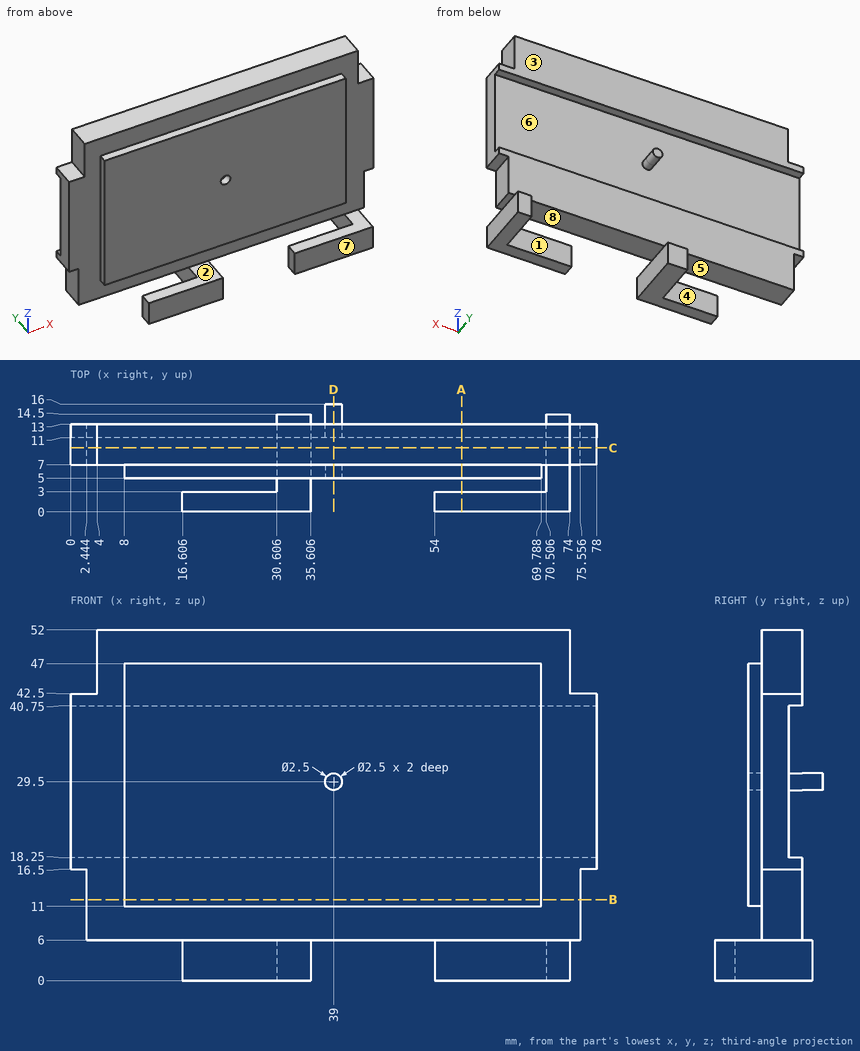
Verification items for this drawing (mm, ordinates from the low corner). A direction names the side the tool comes from. Coordinates: 2 decimals unless noted, no trailing zeros. Write each loop counter-clockwise with the first axis right and the second up, starting at its lowest first coordinate (ties: lowest second). Pieces come first, ordered by that corner, then holes. Notation, with made-up numbers: (-17.5, -0.75) -> (-5.5, -0.75) arc R15 ccw to (-5.5, 21.25) -> close; hole circle Ø11 at (18.5, -36.75). An arc over 180 degrees is marked (long way). One line per item, written item: value. Start each with the question number.
Q1. Cross-section at B-B on z = 12. Enter the section's corners in (x, y) (1 decimal), and give its area (3 significant figures).
Q2. Thickness scan on L1, parallel to Z at x = 54.5, y = 11.25; L2, parallel to Z at x = 39, y = 5.8; L3, parallel to Z at x = 58, y = 6. Record the ranges inside material, lowest first. Write a range as from..to.
Q3. Access from +Z, -Z, +X, -X, +Y, -Y to the whole of each face (thin tool, end or side, straight path). Record for the marked faces 1, 2, 3, 4 and 5.
Q4. Cross-section at D-D on x = 39. Enter the section's corners in (y, z).
Q5. Mould release check, pull along Z, two halves, no side actions. Record for the marked faces 6, 7 and 8: pulls with the +Z half, pulls with the -Z half, needs draft (parallel to the pull), parting line crosses it, or undercut.
Q6. Cross-section at A-A on x = 58. Enter the section's corners in (y, z).
Q7. Cross-section at C-C on y = 9.5. Enter the section's corners in (x, z) (1 decimal), and give its area (3 significant figures).
Q8. Go/stop test with flat-tipped pins: P1, Ø1.5, axis at y = 3.5, z = 28.5, coming from the +X side; P2, Ø1.7, axis at x = 73, z = 2, coming from the +Y side; P3, Ø6.5, axis at y = 9, z = 2.5, coming from the -X side; P4, Ø5, axis at y = 10, z = 47.5, coming from the -X side. Record where each tip stops, or that it passes through.
Checked values:
1. outline: (2.4, 7) -> (8, 7) -> (8, 5) -> (69.8, 5) -> (69.8, 7) -> (75.6, 7) -> (75.6, 13) -> (2.4, 13) -> close
1. area: 562 mm²
2. L1: z = 6..18.25, 40.75..52
2. L2: z = 11..28.25, 30.75..47
2. L3: z = 11..47
3. face 1: +Z, -Z, +Y
3. face 2: +X, -X, -Y
3. face 3: +Z, +X, -X, +Y
3. face 4: +Z, -Z, -X, +Y
3. face 5: -Z, -X, +Y
4. outline: (5, 11) -> (7, 11) -> (7, 6) -> (13, 6) -> (13, 18.25) -> (11, 18.25) -> (11, 28.25) -> (16, 28.25) -> (16, 30.75) -> (11, 30.75) -> (11, 40.75) -> (13, 40.75) -> (13, 52) -> (7, 52) -> (7, 47) -> (5, 47) -> (5, 30.75) -> (7, 30.75) -> (7, 28.25) -> (5, 28.25) -> close
5. face 6: undercut
5. face 7: needs draft
5. face 8: pulls with the -Z half
6. outline: (0, 0) -> (3, 0) -> (3, 6) -> (0, 6) -> close; (5, 11) -> (7, 11) -> (7, 6) -> (13, 6) -> (13, 18.25) -> (11, 18.25) -> (11, 40.75) -> (13, 40.75) -> (13, 52) -> (7, 52) -> (7, 47) -> (5, 47) -> close
7. outline: (0, 16.5) -> (2.4, 16.5) -> (2.4, 6) -> (30.6, 6) -> (30.6, 0) -> (35.6, 0) -> (35.6, 6) -> (70.5, 6) -> (70.5, 0) -> (74, 0) -> (74, 6) -> (75.6, 6) -> (75.6, 16.5) -> (78, 16.5) -> (78, 42.5) -> (74, 42.5) -> (74, 52) -> (4, 52) -> (4, 42.5) -> (0, 42.5) -> close
7. area: 3,510 mm²
8. P1: passes through
8. P2: stops at y = 14.5
8. P3: stops at x = 30.61
8. P4: stops at x = 4
